from build123d import *

# Parameters (mm, degrees)
F0_W     = 25
F0_H     = 20
F1_DEPTH = 19
F2_W     = 25
F2_H     = 6
F3_DEPTH = 2
F5_DEPTH = 19.001


with BuildPart() as f1:
    # F0 (on Front) → F1 (new body)
    with BuildSketch(Plane.XZ):
        Rectangle(F0_W, F0_H)
    extrude(amount=-F1_DEPTH)

    # F2 (on face) → F3 (cut)
    with BuildSketch(Plane.XZ):
        Rectangle(F2_W, F2_H)
    extrude(amount=-F3_DEPTH, mode=Mode.SUBTRACT)

    # F4 (on face) → F5 (cut, through all)
    with BuildSketch(Plane.XZ):
        Polygon((-11.5, 8), (-12.5, 8), (-12.5, 5), (-11.5, 5), (-11.5, 4), (-10.5, 4), (-10.5, 9), (-11.5, 9), align=None)
        Polygon((11.5, 8), (11.5, 9), (10.5, 9), (10.5, 4), (11.5, 4), (11.5, 5), (12.5, 5), (12.5, 8), align=None)
        Polygon((-11.5, -4), (-11.5, -5), (-12.5, -5), (-12.5, -8), (-11.5, -8), (-11.5, -9), (-10.5, -9), (-10.5, -4), align=None)
        Polygon((12.5, -5), (11.5, -5), (11.5, -4), (10.5, -4), (10.5, -9), (11.5, -9), (11.5, -8), (12.5, -8), align=None)
    extrude(amount=-F5_DEPTH, mode=Mode.SUBTRACT)


solid = f1.part
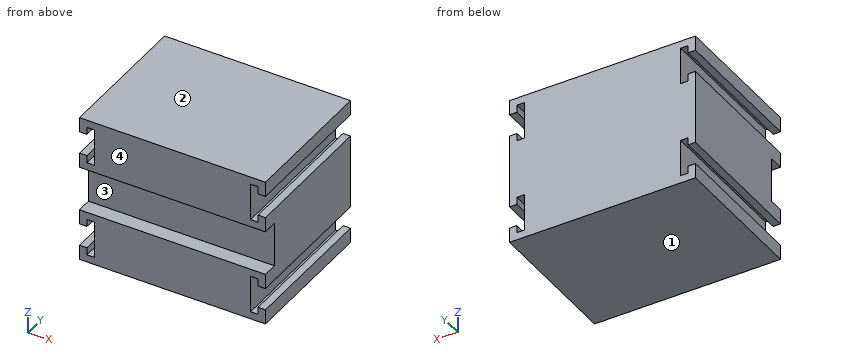
Verification items for the finished model (mm, model axes). Face numbers are marked on the shaded views. Give positions to 0.01 mm unless a question says otherwise; leave off trailing zeros. Loops run counter-clockwise (first coordinate to the right, second up) from the corner with the lowest first, then second, coordinate; pieces in that order, holes last.
1. Release check for a two-part mould opening along Z. For the marked faces 1, 2, 3 and 4 record: +Z half, -Z half, draft (parallel to the pull), parting line (faces both ways), or undercut.
Derived:
face 1: -Z half
face 2: +Z half
face 3: undercut
face 4: draft
2. Go/stop test with a flat-tipped pin: P1, Ø2.5, axis at y = 6.5, z = -7.5, coming from the -X side. Record where the tip stops, or that it passes through.
Derived:
P1: stops at x = -12.5
3. Cross-section at D-D on z = -5.5. Record the cut outline in (x, y).
Derived:
outline: (-10.5, 0) - (10.5, 0) - (10.5, 19) - (-10.5, 19) - close
4. Cross-section at B-B on x = -2.25. Record the cut outline in (y, z).
Derived:
outline: (0, -10) - (19, -10) - (19, 10) - (0, 10) - (0, 3) - (2, 3) - (2, -3) - (0, -3) - close
5. Cross-section at C-C on z = 0. Record the cut outline in (x, y).
Derived:
outline: (-12.5, 2) - (12.5, 2) - (12.5, 19) - (-12.5, 19) - close
6. Cross-section at A-A on z = -8.5. Record the cut outline in (x, y).
Derived:
outline: (-12.5, 0) - (-11.5, 0) - (-11.5, 19) - (-12.5, 19) - close; (-10.5, 0) - (10.5, 0) - (10.5, 19) - (-10.5, 19) - close; (11.5, 0) - (12.5, 0) - (12.5, 19) - (11.5, 19) - close
7. Material ranges on probe 1 along Y at (x, z) = (-10, 1.5); probe 2 along X at (y, z) = (10.25, -6), recorded low to high.
Derived:
probe 1: y = 2 to 19
probe 2: x = -10.5 to 10.5
